Source: CAD feature listing. Evaluate the final solid. Frame: model axes, mm. Round coordinates to 2 decimals unless told otherwise and drop trailing zeros. Loops run counter-clockwise (first coordinate to the right, second up) from the corner with the lowest first, then second, coordinate; pieces in that order, holes last. Notation, with made-up numbers: M 50,0.25 L 57,0.25 A22 cw 57,30.25 Z; hole C 25.25,81.5 d3. An arc over 180 degrees is marked long. Write each question's results on one line, items separated by ' | '. Start each with the question number.
1. Contact query for flat-ended pins moving along their axis: pin 1 Ø5 at (x, z) = (0, 0) entering from -Y; pin 2 Ø5 at (x, z) = (49.5, -2.5) entering from -Y; pin 3 Ø1.5 at (y, z) = (3.5, 3) entering from -X. Output: stop coordinate, or through.
2. Section B-B on y = 1.7. Output: boundary loops of the cut face in (x, z).
3. Ray query, line 1 (Z direction, x = 0, y = 3.6); line 2 (X direction, y = 1.6, z = -1.25); line 3 (X direction, y = 2.05, z = -3). Return the intervals inside material, ascending.
4. Section A-A on z = 0. Output: boundary loops of the cut face in (x, y).
from build123d import *

# Parameters (mm, degrees)
EXTRUDE_1_DEPTH              = 4
HOLE_WIZARD_M5_1_D           = 8
HOLE_WIZARD_M5_1_CBORE_D     = 9.5
HOLE_WIZARD_M5_1_CBORE_DEPTH = 0.9


with BuildPart() as part:
    # 草图1 → 凸台-拉伸1 (new body)
    with BuildSketch(Plane(origin=(0, 0, 0), x_dir=(1, 0, 0), z_dir=(0, 1, 0))):
        with BuildLine():
            Line((0, 6.5), (180, 6.5))
            ThreePointArc((180, 6.5), (186.5, 0), (180, -6.5))
            Line((180, -6.5), (0, -6.5))
            ThreePointArc((0, -6.5), (-6.5, 0), (0, 6.5))
        make_face()
    extrude(amount=EXTRUDE_1_DEPTH)

    # M5 六角头螺栓的柱形沉头孔1 (through all)
    with Locations(Plane(origin=(0, 4, 0), x_dir=(1, 0, 0), z_dir=(0, 1, 0))):
        with Locations((180, 0), (0, 0)):
            CounterBoreHole(HOLE_WIZARD_M5_1_D / 2, HOLE_WIZARD_M5_1_CBORE_D / 2, HOLE_WIZARD_M5_1_CBORE_DEPTH)


solid = part.part
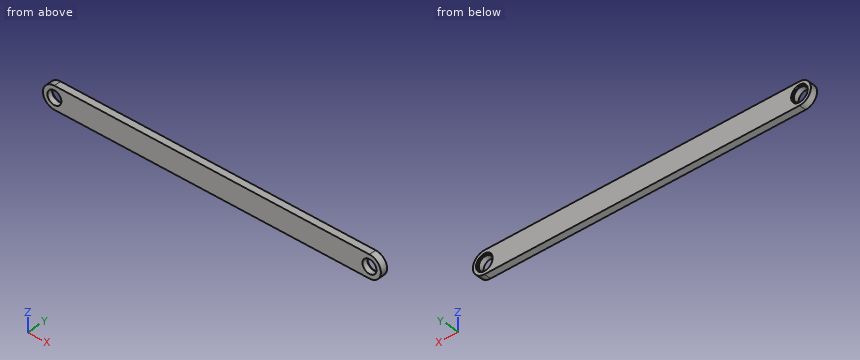
Taken from the geometry:
1) pin 1: through | pin 2: y = 0 | pin 3: x = -6.1
2) outline: M 0,-6.5 L 180,-6.5 A6.5 ccw 180,6.5 L 0,6.5 A6.5 ccw Z; hole C 0,0 d8; hole C 180,0 d8
3) line 1: -6.5 to -4.75, 4.75 to 6.5 | line 2: -6.38 to -3.8, 3.8 to 176.2, 183.8 to 186.38 | line 3: -5.77 to -2.65, 2.65 to 177.35, 182.65 to 185.77
4) outline: M -6.5,0 L -4,0 L -4,3.1 L -4.75,3.1 L -4.75,4 L -6.5,4 Z; M 4,0 L 176,0 L 176,3.1 L 175.25,3.1 L 175.25,4 L 4.75,4 L 4.75,3.1 L 4,3.1 Z; M 184,0 L 186.5,0 L 186.5,4 L 184.75,4 L 184.75,3.1 L 184,3.1 Z
